Verification items for the finished model (mm, model axes). Coordinates: 2 decimals unless noted, no trailing zeros. Order: outer loops, then holes, each group sorted by start corner. A loop starts at its lowest first (then second) coordinate and runs counter-clockwise, first axis right, second up. Notation, with made-up numbers: M 75,53.25 L 122,53.25 A23 cw 122,71.25 Z; hole C 23.25,37 d10. An arc over 180 degrees is marked long. Write item = value, one per line.
```python
from build123d import *

# Parameters (mm, degrees)
SKETCH002_R   = 10
SKETCH002_R_2 = 2.65
PAD002_DEPTH  = 40
PAD003_DEPTH  = 20
CHAMFER_SIZE  = 0.5


with BuildPart() as part:
    # Sketch002 → Pad002 (new body)
    with BuildSketch(Plane.XY):
        Circle(SKETCH002_R)
        Circle(SKETCH002_R_2, mode=Mode.SUBTRACT)
    extrude(amount=PAD002_DEPTH)

    # Sketch003 (on Face3 of Pad002) → Pad003 (join)
    with BuildSketch(Plane(origin=(0, 0, 5), x_dir=(1, 0, 0), z_dir=(0, 0, -1))):
        Polygon((-1.679286, 2.65), (-1.679286, 2.05), (1.679286, 2.05), (1.679286, 2.65), (0, 2.65), align=None)
    extrude(amount=-PAD003_DEPTH)

    # Chamfer
    chamfer_edges = [part.edges().sort_by_distance(p)[0] for p in [
        (0, -2.05, 5),
    ]]
    chamfer(chamfer_edges, length=CHAMFER_SIZE)


solid = part.part
```
Item 1: Sectioned sample at B-B, the plane y = 1. Enter the section's corners in (x, z), then the cut area to 3 significant figures.
Report:
outline = M -9.95,0 L -2.45,0 L -2.45,40 L -9.95,40 Z; M 2.45,0 L 9.95,0 L 9.95,40 L 2.45,40 Z
area = 600 mm^2
Item 2: Sectioned sample at D-D, the plane z = 6. Enter the section's corners in (x, y), then the cut area to 3 significant figures.
Report:
outline = C 0,0 d20; hole M -1.68,-2.05 L 1.68,-2.05 A2.65 ccw long Z
area = 293 mm^2
Item 3: Release check for a two-part mould opening along Y. For faces 1 (the flat face through (0, -2.05, 15)), 2 (the flat face through (2, -2, 0)), 3 (the cylindrical face through (-2.17, -9.76, 19.72)) record: pulls with the +Y half, pulls with the -Y half, needs draft (parallel to the pull), parting line crosses it, or undercut.
Report:
face_1 = undercut
face_2 = needs draft
face_3 = parting line crosses it
Item 4: Gauge pin test, flat ends, axial feed: pin 1 (10 mm diameter, centred on x = 4.5, z = 7.5, fed in from -Y); pin 2 (6 mm diameter, centred on y = -4, z = 18.5, fed in from +X); pin 3 (1 mm diameter, centred on y = 2, z = 23.5, fed in from -X); pin 4 (1 mm diameter, centred on x = -4.5, z = 29, fed in from +Y). Record the tip position at first contact, or that the pin passes through.
Report:
pin_1 = -10
pin_2 = 9.95
pin_3 = -9.89
pin_4 = 9.17
Item 5: Scan lines: L1, parallel to Y at x = 0, z = 29; L2, parallel to Y at x = 0, z = 19.5; L3, parallel to X at y = -1.25, z = 35. Record each from-to range of solid material in increasing order. Write a range as from..to.
Report:
L1 = -10..-2.65, 2.65..10
L2 = -10..-2.05, 2.65..10
L3 = -9.92..-2.34, 2.34..9.92
Item 6: Sectioned sample at A-A, the plane x = 0. Enter the section's corners in (y, z).
Report:
outline = M -10,0 L -2.65,0 L -2.65,5 L -2.55,5 L -2.05,5.5 L -2.05,25 L -2.65,25 L -2.65,40 L -10,40 Z; M 2.65,0 L 10,0 L 10,40 L 2.65,40 Z
Item 7: Sectioned sample at C-C, the plane z = 35.5. Enter the section's corners in (x, y).
Report:
outline = C 0,0 d20; hole C 0,0 d5.3
